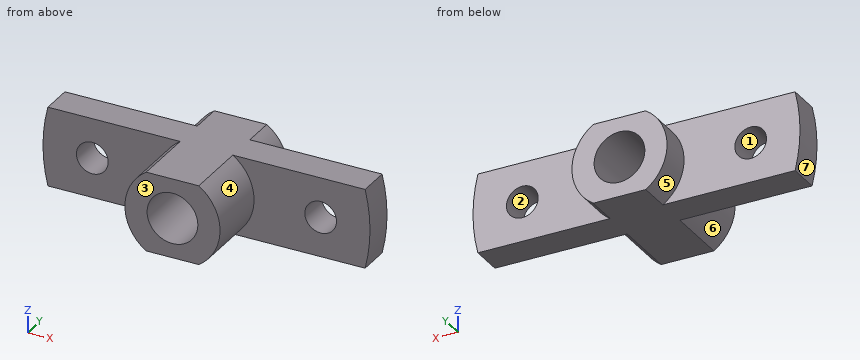
```python
from build123d import *

# Parameters (mm, degrees)
F1_DEPTH      = 30
F1_DEPTH_BACK = 10
F0_R          = 5
F2_DEPTH      = 10


with BuildPart() as f1:
    # F0 (on Front) → F1 (new body, two sides)
    with BuildSketch(Plane.XZ) as f1_sk:
        with BuildLine():
            ThreePointArc((0, 8), (8, 0), (0, -8))
            Line((0, -8), (0, -12.5))
            Line((0, -12.5), (8.291562, -12.5))
            ThreePointArc((8.291562, -12.5), (15, 0), (8.291562, 12.5))
            Line((8.291562, 12.5), (0, 12.5))
            Line((0, 12.5), (0, 8))
        make_face()
    extrude(amount=F1_DEPTH)
    extrude(f1_sk.sketch, amount=-F1_DEPTH_BACK)

    # F0 (on Front) → F2 (join)
    with BuildSketch(Plane.XZ):
        with BuildLine():
            ThreePointArc((8.291562, 12.5), (15, 0), (8.291562, -12.5))
            Line((8.291562, -12.5), (50, -12.5))
            ThreePointArc((50, -12.5), (51.53882, 0), (50, 12.5))
            Line((50, 12.5), (8.291562, 12.5))
        make_face()
        with Locations((36, 0)):
            Circle(F0_R, mode=Mode.SUBTRACT)
    extrude(amount=F2_DEPTH)

    # F3: F1 across plane


with BuildPart() as f1_1:
    add(f1.part)
    add(f1.part.mirror(Plane.YZ))


solid = f1_1.part
```
Geometry check sheet. Reference: the model listing, model coordinates, mm. Face numbers are marked on the shaded views. A direction names the side the tool comes from. Round coordinates to 2 decimals unless told otherwise and drop trailing zeros. Loops run counter-clockwise (first coordinate to the right, second up) from the corner with the lowest first, then second, coordinate; pieces in that order, holes last. Notation, with made-up numbers: M -26,48 L 14,48 A26 ccw 14,63 Z; hole C 70,11 d3. An arc over 180 degrees is marked long. Return JSON: item names as keys, results as strings. Group by question number.
(1) Set-up check for the marked faces 5, 6 and 7: record each of +Z, -Z, +X, -X, +Y, -Y from which the full face is reachable in a straight line by a thin tool's end or side.
(2) Section check B-B, the plane z = 0. Enter the section's corners in (x, y).
(3) Section check D-D, the plane x = -36. Enter the section's corners in (y, z), and give its area (3 significant figures).
(4) Section check A-A, the plane x = 0. Enter the section's corners in (y, z), and give its area (3 significant figures).
(5) Mould release check, pull along X, two halves, no side actions. Record for the marked faces 1, 2, 3 and 4: pulls with the +X half, pulls with the -X half, needs draft (parallel to the pull), parting line crosses it, or undercut.
(6) Scan lines: line 1 along Z through (x, y) = (-36, -5); line 2 along Z through (x, y) = (0, -20); line 3 along Y through (x, z) = (15, -3). Record each from-to range of solid material in increasing order. Write a range as [from, to].
(7) Section check C-C, the plane y = -14. Enter the section's corners in (x, z), and give its area (3 significant figures).
(8) Go/stop test with flat-tipped pins: pin 1 (1 mm diameter, centred on y = -26, z = -4, fed in from +X); pin 2 (7.5 mm diameter, centred on x = 20, z = 6, fed in from +Y); pin 3 (5 mm diameter, centred on x = 24.5, z = -9.5, fed in from -Y); pin 4 (12 mm diameter, centred on x = 34.5, y = -11, fed in from -Z). Record where each tip stops, or that it passes through.
Data:
{
 "1": {"face 5": "-X, +Y", "face 6": "-X, -Y", "face 7": "-X, +Y, -Y"},
 "2": {"outline": "M -51.54,-10 L -41,-10 L -41,0 L -51.54,0 Z; M -31,-10 L -15,-10 L -15,-30 L -8,-30 L -8,10 L -15,10 L -15,0 L -31,0 Z; M 8,-30 L 15,-30 L 15,-10 L 31,-10 L 31,0 L 15,0 L 15,10 L 8,10 Z; M 41,-10 L 51.54,-10 L 51.54,0 L 41,0 Z"},
 "3": {"outline": "M -10,-12.5 L 0,-12.5 L 0,-5 L -10,-5 Z; M -10,5 L 0,5 L 0,12.5 L -10,12.5 Z", "area": "150 mm²"},
 "4": {"outline": "M -30,-12.5 L 10,-12.5 L 10,-8 L -30,-8 Z; M -30,8 L 10,8 L 10,12.5 L -30,12.5 Z", "area": "360 mm²"},
 "5": {"face 1": "undercut", "face 2": "undercut", "face 3": "needs draft", "face 4": "pulls with the +X half"},
 "6": {"line 1": "[-12.5, -5], [5, 12.5]", "line 2": "[-12.5, -8], [8, 12.5]", "line 3": "[-10, 0]"},
 "7": {"outline": "M -8.29,-12.5 L 8.29,-12.5 A15 ccw 8.29,12.5 L -8.29,12.5 A15 ccw Z; hole C 0,0 d16", "area": "450 mm²"},
 "8": {"pin 1": "x = 14.59", "pin 2": "y = 0", "pin 3": "y = -10", "pin 4": "z = -12.5"}
}
